Input: part model. Units: mm. Frame: model coordinates. A direction names the side the tool comes from. Give positions to 0.01 mm unless a question says otherwise; leave off trailing zeros. Loops run counter-clockwise (first coordinate to the right, second up) from the corner with the lowest first, then second, coordinate; pieces in that order, holes last. Notation, with made-up numbers: (-0.75, 44) - (55.25, 44) arc R16 ccw to (55.25, 61) - close; hole circle Ø6 at (-3, 65). An arc over 180 degrees is marked (long way). Answer as a JSON object with one key per item and string values.
Autodesk Inventor part; units mm, degrees
ref_plane "YZ Plane" through (0, 0, 0) normal (1, 0, 0) x (0, 1, 0)
ref_plane "XZ Plane" through (0, 0, 0) normal (0, 1, 0) x (-1, 0, 0)
ref_plane "XY Plane" through (0, 0, 0) normal (0, 0, 1) x (1, 0, 0)
sketch "Skizze1" plane through (0, 0, 0) normal (0, 1, 0) x (-1, 0, 0)
  line L0 (23.4402, 37.0701) -> (-56.5598, 37.0701)
  line L1 (-56.5598, 37.0701) -> (-56.5598, -38.9299)
  line L2 (-56.5598, -38.9299) -> (23.4402, -38.9299)
  line L3 (23.4402, -38.9299) -> (23.4402, 37.0701)
  point P0 (0, 0)
  dimension "d0" = 76
  dimension "d1" = 80
extrude "Extrusion1" add sketch "Skizze1" along normal blind 6
sketch "Skizze8" plane through (0, 0, 0) normal (0, -1, 0) x (1, 0, 0)
  line L0 (47.5598, 24.0701) -> (47.5598, -25.9299) construction
  line L1 (49.0598, 24.0701) -> (49.0598, -25.9299)
  line L2 (46.0598, -25.9299) -> (46.0598, 24.0701)
  arc A0 (49.0598, 24.0701) -> (46.0598, 24.0701) centre (47.5598, 24.0701) ccw
  arc A1 (46.0598, -25.9299) -> (49.0598, -25.9299) centre (47.5598, -25.9299) ccw
  line L3 (52.5598, -0.9299) -> (-23.4402, -0.9299)
  line L4 (39.5598, 24.0701) -> (39.5598, -25.9299) construction
  line L5 (38.0598, 24.0701) -> (38.0598, -25.9299)
  line L6 (41.0598, -25.9299) -> (41.0598, 24.0701)
  arc A2 (41.0598, 24.0701) -> (38.0598, 24.0701) centre (39.5598, 24.0701) ccw
  arc A3 (38.0598, -25.9299) -> (41.0598, -25.9299) centre (39.5598, -25.9299) ccw
  line L7 (56.5598, 37.0701) -> (56.5598, -38.9299)
  line L8 (56.5598, -38.9299) -> (-23.4402, -38.9299)
  line L9 (41.0598, 24.0701) -> (38.0598, 24.0701) construction
  line L10 (41.0598, -25.9299) -> (38.0598, -25.9299) construction
  line L11 (49.0598, -25.9299) -> (46.0598, -25.9299) construction
  arc A4 (30.0598, -25.9299) -> (33.0598, -25.9299) centre (31.5598, -25.9299) ccw
  line L12 (31.5598, 24.0701) -> (31.5598, -25.9299) construction
  line L13 (30.0598, 24.0701) -> (30.0598, -25.9299)
  line L14 (33.0598, -25.9299) -> (33.0598, 24.0701)
  arc A5 (33.0598, 24.0701) -> (30.0598, 24.0701) centre (31.5598, 24.0701) ccw
  line L15 (33.0598, 24.0701) -> (30.0598, 24.0701) construction
  line L16 (33.0598, -25.9299) -> (30.0598, -25.9299) construction
  line L17 (25.0598, 24.0701) -> (22.0598, 24.0701) construction
  arc A6 (25.0598, 24.0701) -> (22.0598, 24.0701) centre (23.5598, 24.0701) ccw
  line L18 (25.0598, -25.9299) -> (25.0598, 24.0701)
  line L19 (23.5598, 24.0701) -> (23.5598, -25.9299) construction
  line L20 (22.0598, 24.0701) -> (22.0598, -25.9299)
  line L21 (25.0598, -25.9299) -> (22.0598, -25.9299) construction
  arc A7 (22.0598, -25.9299) -> (25.0598, -25.9299) centre (23.5598, -25.9299) ccw
  line L22 (-23.4402, 37.0701) -> (56.5598, 37.0701)
  line L23 (-23.4402, -38.9299) -> (-23.4402, 37.0701)
  circle A8 centre (-4.9402, -20.4299) radius 10.5
  point P0 (47.5598, -0.9299)
  point P1 (35.0598, -0.9299)
  dimension "d69" = 7.5
  dimension "d70" = 50
  dimension "d71" = 38
  dimension "d72" = 5
  dimension "d74" = 3
  dimension "d75" = 5
  dimension "d76" = 5
  dimension "d109" = 21
  dimension "d110" = 18.5
  dimension "d111" = 18.5
extrude "Extrusion8" cut sketch "Skizze8" against normal blind 10 contours L18 A7 L20 L3 | L3 L20 A6 L18 | L14 A4 L13 L3 | L3 L13 A5 L14 | L6 A3 L5 L3 | L3 L5 A2 L6 | L1 L3 L2 A0 | L1 A1 L2 L3 | A8
sketch "Skizze14" plane through (0, 6, 0) normal (0, 1, 0) x (1, 0, 0)
  line L0 (-20.7402, -34.3701) -> (-14.7402, -34.3701)
  line L1 (-14.7402, -34.3701) -> (-14.7402, -28.3701)
  line L2 (-14.7402, -28.3701) -> (-20.7402, -28.3701)
  line L3 (-20.7402, -28.3701) -> (-20.7402, -34.3701)
  line L4 (-20.7402, 36.2299) -> (-14.7402, 36.2299)
  line L5 (-14.7402, 36.2299) -> (-14.7402, 30.2299)
  line L6 (-14.7402, 30.2299) -> (-20.7402, 30.2299)
  line L7 (-20.7402, 30.2299) -> (-20.7402, 36.2299)
  line L8 (-23.4402, 38.9299) -> (-23.4402, -37.0701)
  line L9 (56.5598, 38.9299) -> (-23.4402, 38.9299)
  line L10 (-23.4402, -37.0701) -> (56.5598, -37.0701)
  line L11 (47.8598, 30.2299) -> (53.8598, 30.2299)
  line L12 (53.8598, 30.2299) -> (53.8598, 36.2299)
  line L13 (53.8598, 36.2299) -> (47.8598, 36.2299)
  line L14 (47.8598, 36.2299) -> (47.8598, 30.2299)
  line L15 (53.8598, -34.3701) -> (47.8598, -34.3701)
  line L16 (47.8598, -34.3701) -> (47.8598, -28.3701)
  line L17 (47.8598, -28.3701) -> (53.8598, -28.3701)
  line L18 (53.8598, -28.3701) -> (53.8598, -34.3701)
  line L19 (56.5598, -37.0701) -> (56.5598, 38.9299)
  point P0 (0, 0)
  dimension "d83" = 6
  dimension "d84" = 2.7
  dimension "d85" = 2.7
  dimension "d86" = 2.7
  dimension "d112" = 2.7
extrude "Extrusion14" add sketch "Skizze14" along normal blind 6.5 contours L3 L2 L1 L0 | L4 L5 L6 L7 | L14 L13 L12 L11 | L15 L16 L17 L18
sketch "Skizze17" plane through (-20.7402, 6, -36.2299) normal (-1, 0, 0) x (0, 0, 1)
  circle A0 centre (67.6, 3.25) radius 0.75
  circle A1 centre (3, 3.25) radius 0.75
  line L0 (-2.7, 0) -> (73.3, 0)
  line L1 (0, 0) -> (0, 6.5)
  line L2 (70.6, 0) -> (70.6, 6.5)
  point P0 (36.2299, -6)
  dimension "d102" = 3.25
  dimension "d103" = 1.5
  dimension "d104" = 3
  dimension "d105" = 3
  dimension "d106" = 3.25
extrude "Extrusion17" cut sketch "Skizze17" against normal through all
chamfer "Fase1" distance 2 angle 45 4 edges at (-14.7402, 9.25, 28.3701) (-14.7402, 9.25, -30.2299) (47.8598, 9.25, 28.3701) (47.8598, 9.25, -30.2299)
properties part number "cover without shutdown button"
Item 1: Cut plane A-A (z = -3.5). Return loops of the section in (x, y).
Geometry check:
{"outline": "(-23.44, 0) - (22.06, 0) - (22.06, 6) - (-23.44, 6) - close; (25.06, 0) - (30.06, 0) - (30.06, 6) - (25.06, 6) - close; (33.06, 0) - (38.06, 0) - (38.06, 6) - (33.06, 6) - close; (41.06, 0) - (46.06, 0) - (46.06, 6) - (41.06, 6) - close; (49.06, 0) - (56.56, 0) - (56.56, 6) - (49.06, 6) - close"}
Item 2: Contact query for flat-ended pins moving along their axis: P1, Ø1.2, axis at y = 9.25, z = 31.37, coming from the +X side; P2, Ø1.2, axis at y = 9, z = 32.5, coming from the -X side; P3, Ø4, axis at x = -9, z = 9, coming from the +Y side; P4, Ø3, axis at y = 8, z = 32.5, coming from the +X side. Output: stop coordinate, or through.
Geometry check:
{"P1": "passes through", "P2": "stops at x = -20.74", "P3": "stops at y = 6", "P4": "stops at x = 53.86"}
Item 3: Material intervals for line 1 (X direction, y = 0.5, z = -9); line 2 (X direction, y = 0.5, z = -21); line 3 (X direction, y = 5.5, z = -15), sorted ascending. Write a range as [from, to].
Geometry check:
{"line 1": "x = [-23.44, 22.06], [25.06, 30.06], [33.06, 38.06], [41.06, 46.06], [49.06, 56.56]", "line 2": "x = [-23.44, -15.42], [5.54, 22.06], [25.06, 30.06], [33.06, 38.06], [41.06, 46.06], [49.06, 56.56]", "line 3": "x = [-23.44, -13.93], [4.05, 22.06], [25.06, 30.06], [33.06, 38.06], [41.06, 46.06], [49.06, 56.56]"}
Item 4: Cut plane C-C (y = 3.5). Return loops of the section in (x, z), then the cut area to 3 significant figures.
Geometry check:
{"outline": "(-23.44, -38.93) - (56.56, -38.93) - (56.56, 37.07) - (-23.44, 37.07) - close; hole circle Ø21 at (-4.94, -20.43); hole (22.06, -25.93) arc R1.5 ccw to (25.06, -25.93) - (25.06, 24.07) arc R1.5 ccw to (22.06, 24.07) - close; hole (30.06, -25.93) arc R1.5 ccw to (33.06, -25.93) - (33.06, 24.07) arc R1.5 ccw to (30.06, 24.07) - close; hole (38.06, -25.93) arc R1.5 ccw to (41.06, -25.93) - (41.06, 24.07) arc R1.5 ccw to (38.06, 24.07) - close; hole (46.06, -25.93) arc R1.5 ccw to (49.06, -25.93) - (49.06, 24.07) arc R1.5 ccw to (46.06, 24.07) - close", "area": "5,110 mm2"}
Item 5: Cut plane B-B (x = -1). Return loops of the section in (y, z).
Geometry check:
{"outline": "(0, -38.93) - (6, -38.93) - (6, -30.16) - (0, -30.16) - close; (0, -10.7) - (6, -10.7) - (6, 37.07) - (0, 37.07) - close"}
Item 6: Mould query, pull axis Z, two halves, no side actions, for faces 6 (the face through (51, 9, -36.23)), 7 (the face through (-18, 12.5, 31)), 8 (the face through (-18, 9, 34.37)), 9 (the face through (31.59, 2.96, 25.57)). Classes: released by +Z, released by -Z, zero draft, split by the parting line, or undercut.
Geometry check:
{"face 6": "released by -Z", "face 7": "zero draft", "face 8": "released by +Z", "face 9": "undercut"}
Item 7: Access query for faces 1 (the face through (-15.75, 9.3, 29.36)), 2 (the face through (51, 12.5, -33)), 3 (the face through (47.86, 9.2, 32.4)), 4 (the face through (-19, 9, -30.23)), 5 (the face through (25.06, 3, -1)). Directions: +Z, -Z, +X, -X, +Y, -Y. A direction counts if a zero-diameter tool reaches every point of the face in a straight line with its end or side. Return the directions, or none.
Geometry check:
{"face 1": "+Y", "face 2": "+Z, -Z, +X, -X, +Y", "face 3": "+Z, -Z, +Y", "face 4": "+X, -X, +Y", "face 5": "+Y, -Y"}
Item 8: Cut plane D-D (x = 15.5). Return loops of the section in (y, z).
Geometry check:
{"outline": "(0, -38.93) - (6, -38.93) - (6, 37.07) - (0, 37.07) - close"}
